The listing builds one solid part. Answer for the finished solid, in the listing's coordinates (mm). Face numbers are marked on the shaded views. A direction names the side the tool comes from. Round coordinates to 2 decimals unless told otherwise and drop trailing zeros. Write each loop counter-clockwise with the first axis right and the second up, starting at its lowest first coordinate (ties: lowest second). Pieces come first, ordered by that corner, then holes. Notation, with made-up numbers: (4, 83.25) - (8, 83.25) arc R9 ccw to (8, 99.25) - close; hole circle Ø5 at (59, 87). An arc over 180 degrees is marked (long way). Use a Markdown table: item, result. Add a question column.
1) A cutting plane is placed at B-B (y = 0). Give the vertices of the cut face in (x, z).
2) Find the intervals of material crossed by probe 1 along X at (y, z) = (0, -4.95); probe 2 along X at (y, z) = (0, -1.7); probe 3 along X at (y, z) = (-26.5, -2.75), in increasing order. Write a range as from..to.
3) A cutting plane is placed at A-A (z = 3.5). Give the vertices of the cut face in (x, y), then the cut area to 3 significant figures.
4) A cutting plane is placed at C-C (y = -26.5). Give the vertices of the cut face in (x, z), then the cut area to 3 significant figures.
5) Each of these flat-tipped pins is pushed along its axis until it touches: P1, Ø13.5, axis at x = 6.9, y = 0, coming from the +Z side; P2, Ø7, axis at x = -6.905, y = 0, coming from the -Z side; P3, Ø10, axis at x = 6.9, y = 0, coming from the +Z side. Where does it stop, or does it pass through?
6) Determine the mould class of the marked faces 1, 2 and 3 for opening direction X: +X half, -X half, draft (parallel to the pull), parting line (faces both ways), or undercut.
7) A cutting plane is placed at D-D (z = -5). Give the vertices of the cut face in (x, y) (1 decimal), then the cut area to 3 significant figures.
8) A tool of negligible diameter and unlimited length cuts with its end or side. For the marked faces 4, 5 and 6, from which of +Z, -Z, +X, -X, +Y, -Y can it reach the whole face along a straight path? Write none if from no direction.
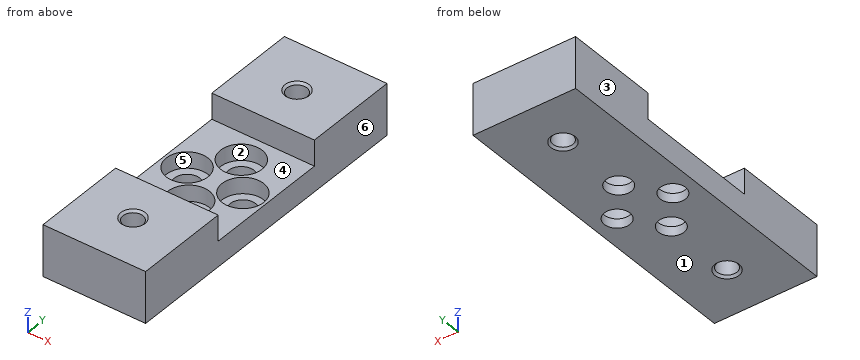
Autodesk Inventor part; units mm, degrees
ref_plane "screw1_XY" through (-6.905, 0, -4.0132) normal (0, 0, 1) x (1, 0, 0)
ref_plane "screw1_YZ" through (-6.905, 0, -4.0132) normal (1, 0, 0) x (0, 1, 0)
ref_plane "screw1_ZX" through (-6.905, 0, -4.0132) normal (0, 1, 0) x (0, 0, 1)
sketch "Sketch_1" plane through (0, 0, 0) normal (1, 0, 0) x (0, 1, 0)
  line L0 (-15.55, 6.4) -> (-39, 6.4)
  line L1 (-39, 6.4) -> (-39, -6.3)
  line L2 (-39, -6.3) -> (39, -6.3)
  line L3 (39, -6.3) -> (39, 6.4)
  line L4 (39, 6.4) -> (15.55, 6.4)
  line L5 (15.55, 6.4) -> (15.55, 0)
  line L6 (15.55, 0) -> (-15.55, 0)
  line L7 (-15.55, 0) -> (-15.55, 6.4)
extrude "Extrusion1" add sketch "Sketch_1" along normal mid plane 25.4
sketch "Sketch_2" plane through (0, 0, 0) normal (1, 0, 0) x (0, 1, 0)
  line L0 (26.5, -6.3) -> (26.5, 6.4)
  line L1 (26.5, 6.4) -> (29.5, 6.4)
  line L2 (29.5, 6.4) -> (28.9585, 5.8585)
  line L3 (28.9585, 5.8585) -> (28.9585, -5.7585)
  line L4 (28.9585, -5.7585) -> (29.5, -6.3)
  line L5 (29.5, -6.3) -> (26.5, -6.3)
  line L6 (26.5, -6.3) -> (26.5, 6.4)
revolve "Revolution1" cut sketch "Sketch_2" angle 360 about axis through (0, 26.5, -6.3) along (0, 0, -1)
thread "Thread1"
sketch "Sketch_3" plane through (0, 0, 0) normal (1, 0, 0) x (0, 1, 0)
  line L0 (-26.5, -6.3) -> (-26.5, 6.4)
  line L1 (-26.5, 6.4) -> (-23.5, 6.4)
  line L2 (-23.5, 6.4) -> (-24.0415, 5.8585)
  line L3 (-24.0415, 5.8585) -> (-24.0415, -5.7585)
  line L4 (-24.0415, -5.7585) -> (-23.5, -6.3)
  line L5 (-23.5, -6.3) -> (-26.5, -6.3)
  line L6 (-26.5, -6.3) -> (-26.5, 6.4)
revolve "Revolution2" cut sketch "Sketch_3" angle 360 about axis through (0, -26.5, -6.3) along (0, 0, -1)
thread "Thread2"
sketch "Sketch4" plane through (-12.7, -15.55, 0) normal (0, 0, 1) x (1, 0, 0)
  point P0 (5.795, 15.55)
hole "Hole1" at (-6.905, 0, 0) direction (0, 0, -1) diameter 6.2992 depth 6.3 counterbore diameter 10.3124 counterbore depth 4.0132
pattern_linear "Rectangular Pattern1" count 2 spacing 10.9512 along (0.6305, 0.7762, 0) count 2 spacing 10.9512 along (0.6305, -0.7762, 0) of "Hole1"
ref_plane "screw1_XY" through (-6.905, 0, -4.0132) normal (0, 0, 1) x (1, 0, 0)
ref_plane "screw1_YZ" through (-6.905, 0, -4.0132) normal (1, 0, 0) x (0, 1, 0)
ref_plane "screw1_ZX" through (-6.905, 0, -4.0132) normal (0, 1, 0) x (0, 0, 1)
ref_plane "screw1_1_XY" through (0, 8.5, -4.0132) normal (0, 0, 1) x (1, 0, 0)
ref_plane "screw1_1_YZ" through (0, 8.5, -4.0132) normal (1, 0, 0) x (0, 1, 0)
ref_plane "screw1_1_ZX" through (0, 8.5, -4.0132) normal (0, 1, 0) x (0, 0, 1)
ref_plane "screw2_XY" through (6.905, 0, -4.0132) normal (0, 0, 1) x (1, 0, 0)
ref_plane "screw2_YZ" through (6.905, 0, -4.0132) normal (1, 0, 0) x (0, 1, 0)
ref_plane "screw2_ZX" through (6.905, 0, -4.0132) normal (0, 1, 0) x (0, 0, 1)
ref_plane "screw2_1_XY" through (0, -8.5, -4.0132) normal (0, 0, 1) x (1, 0, 0)
ref_plane "screw2_1_YZ" through (0, -8.5, -4.0132) normal (1, 0, 0) x (0, 1, 0)
ref_plane "screw2_1_ZX" through (0, -8.5, -4.0132) normal (0, 1, 0) x (0, 0, 1)
ref_plane "to_dummy_XY" through (0, 0, 0) normal (0, 0, 1) x (1, 0, 0)
ref_plane "to_dummy_YZ" through (0, 0, 0) normal (1, 0, 0) x (0, 1, 0)
ref_plane "to_dummy_ZX" through (0, 0, 0) normal (0, 1, 0) x (0, 0, 1)
ref_plane "to_wheel1_XY" through (0, 26.5, 6.4) normal (0, 0, 1) x (1, 0, 0)
ref_plane "to_wheel1_YZ" through (0, 26.5, 6.4) normal (1, 0, 0) x (0, 1, 0)
ref_plane "to_wheel1_ZX" through (0, 26.5, 6.4) normal (0, 1, 0) x (0, 0, 1)
ref_plane "to_wheel2_XY" through (0, -26.5, 6.4) normal (0, 0, 1) x (1, 0, 0)
ref_plane "to_wheel2_YZ" through (0, -26.5, 6.4) normal (1, 0, 0) x (0, 1, 0)
ref_plane "to_wheel2_ZX" through (0, -26.5, 6.4) normal (0, 1, 0) x (0, 0, 1)
properties part number "25-2750-1_p"
Entries:
| question | item | result |
|---|---|---|
| 1 | outline | (-12.7, -6.3) - (-10.05, -6.3) - (-10.05, -4.01) - (-12.06, -4.01) - (-12.06, 0) - (-12.7, 0) - close; (-3.76, -6.3) - (3.75, -6.3) - (3.75, -4.01) - (1.75, -4.01) - (1.75, 0) - (-1.75, 0) - (-1.75, -4.01) - (-3.76, -4.01) - close; (10.05, -6.3) - (12.7, -6.3) - (12.7, 0) - (12.06, 0) - (12.06, -4.01) - (10.05, -4.01) - close |
| 2 | probe 1 | x = -12.7..-10.05, -3.76..3.75, 10.05..12.7 |
| 2 | probe 2 | x = -12.7..-12.06, -1.75..1.75, 12.06..12.7 |
| 2 | probe 3 | x = -12.7..-2.46, 2.46..12.7 |
| 3 | outline | (-12.7, -39) - (12.7, -39) - (12.7, -15.55) - (-12.7, -15.55) - close; (-12.7, 15.55) - (12.7, 15.55) - (12.7, 39) - (-12.7, 39) - close; hole circle Ø4.92 at (0, -26.5); hole circle Ø4.92 at (0, 26.5) |
| 3 | area | 1,150 mm² |
| 4 | outline | (-12.7, -6.3) - (-3, -6.3) - (-2.46, -5.76) - (-2.46, 5.86) - (-3, 6.4) - (-12.7, 6.4) - close; (2.46, -5.76) - (3, -6.3) - (12.7, -6.3) - (12.7, 6.4) - (3, 6.4) - (2.46, 5.86) - close |
| 4 | area | 260 mm² |
| 5 | P1 | stops at z = 0 |
| 5 | P2 | stops at z = -6.3 |
| 5 | P3 | stops at z = -4.01 |
| 6 | face 1 | draft |
| 6 | face 2 | undercut |
| 6 | face 3 | -X half |
| 7 | outline | (-12.7, -39) - (12.7, -39) - (12.7, 39) - (-12.7, 39) - close; hole circle Ø6.3 at (-6.9, 0); hole circle Ø6.3 at (0, -8.5); hole circle Ø6.3 at (0, 8.5); hole circle Ø4.9 at (0, -26.5); hole circle Ø4.9 at (0, 26.5); hole circle Ø6.3 at (6.9, 0) |
| 7 | area | 1,820 mm² |
| 8 | face 4 | +Z, +X, -X |
| 8 | face 5 | +Z |
| 8 | face 6 | +Z, -Z, +X, +Y, -Y |
